Geometry check sheet. Reference: the model listing, model coordinates, mm. Face numbers are marked on the shaded views. A direction names the side the tool comes from. Round coordinates to 2 decimals unless told otherwise and drop trailing zeros. Return JSON: item names as keys, results as strings.
```python
from build123d import *

# Parameters (mm, degrees)
CONG_2_R           = 2
ESQUISSE3_W        = 5
ESQUISSE3_H        = 5
BOSS_EXTRU_1_DEPTH = 10
ESQUISSE4_W        = 6
ESQUISSE4_H        = 6
BOSS_EXTRU_2_DEPTH = 3


with BuildPart() as part:
    # Esquisse1 → Révolution1 (revolve)
    with BuildSketch(Plane.XY):
        with BuildLine():
            Line((0, 0), (12.5, 0))
            add(Edge.make_bspline(
                [(12.5, 0), (-2.792999131, 19.477640693), (36.048194097, 21.903623333), (22, 40)],
                knots=[0, 0, 0, 0, 1, 1, 1, 1], degree=3))
            Line((22, 40), (0, 40))
            Line((0, 40), (0, 0))
        make_face()
    revolve(axis=Axis((0, 0, 0), (0, 1, 0)))

    # Esquisse2 → Enlèvement de matière-Révolution1 (revolve, cut)
    with BuildSketch(Plane.XY):
        with BuildLine():
            Line((-14.44702814, 40), (0, 40))
            Line((0, 40), (0, 37.486983962))
            Line((0, 37.486983962), (-11.204408598, 37.486983962))
            add(Edge.make_bspline(
                [(-14.44702814, 40), (-13.476590785, 37.876911576), (-11.204408598, 37.486983962)],
                knots=[0, 0, 0, 1, 1, 1], degree=2))
        make_face()
    revolve(axis=Axis((0, -3.04576032, 0), (0, 1, 0)), mode=Mode.SUBTRACT)

    # Congé2
    cong_2_edges = [part.edges().sort_by_distance(p)[0] for p in [
        (-22, 40, 0),
    ]]
    fillet(cong_2_edges, radius=CONG_2_R)

    # Esquisse3 → Boss.-Extru.1 (add)
    with BuildSketch(Plane.XZ):
        Rectangle(ESQUISSE3_W, ESQUISSE3_H)
    extrude(amount=BOSS_EXTRU_1_DEPTH)

    # Esquisse4 → Boss.-Extru.2 (add)
    with BuildSketch(Plane.XZ.offset(10)):
        Rectangle(ESQUISSE4_W, ESQUISSE4_H)
    extrude(amount=-BOSS_EXTRU_2_DEPTH)


solid = part.part
```
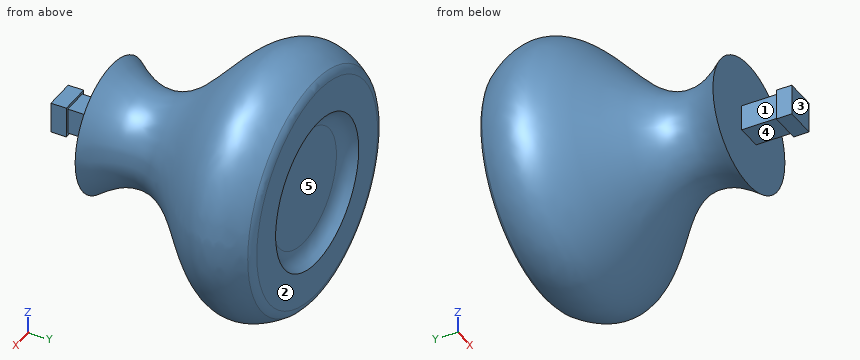
(1) Material ranges on line 1 along X through (y, z) = (-8, 0.5); line 2 along Y through (x, z) = (4.5, -1); line 3 along Y through (x, z) = (-7.5, 8), recorded low to high. Write a range as [from, to].
Response values:
{"line 1": "x = [-3, 3]", "line 2": "y = [0, 37.49]", "line 3": "y = [0, 2.18], [14.57, 37.49]"}
(2) Release check for a two-part mould opening along Y. For the marked faces 1 and 2 record: pulls with the +Y half, pulls with the -Y half, needs draft (parallel to the pull), parting line crosses it, or undercut.
Response values:
{"face 1": "undercut", "face 2": "pulls with the +Y half"}
(3) Gauge pin test, flat ends, axial feed: pin 1 (2.5 mm diameter, centred on x = -0.5, y = -3.5, fed in from -Z); pin 2 (1.5 mm diameter, centred on y = -4.5, z = 1, fed in from +X); pin 3 (12 mm diameter, centred on x = 1, z = -6, fed in from +Y). Record the tip position at first contact, or that the pin passes through.
Response values:
{"pin 1": "stops at z = -2.5", "pin 2": "stops at x = 2.5", "pin 3": "stops at y = 37.72"}
(4) Access from +Z, -Z, +X, -X, +Y, -Y to the whole of each face (thin tool, end or side, straight path). Record for the marked faces 3, 4 and 5.
Response values:
{"face 3": "+Z, -Z, +X, -X, -Y", "face 4": "-Z, +X, -X", "face 5": "+Y"}
